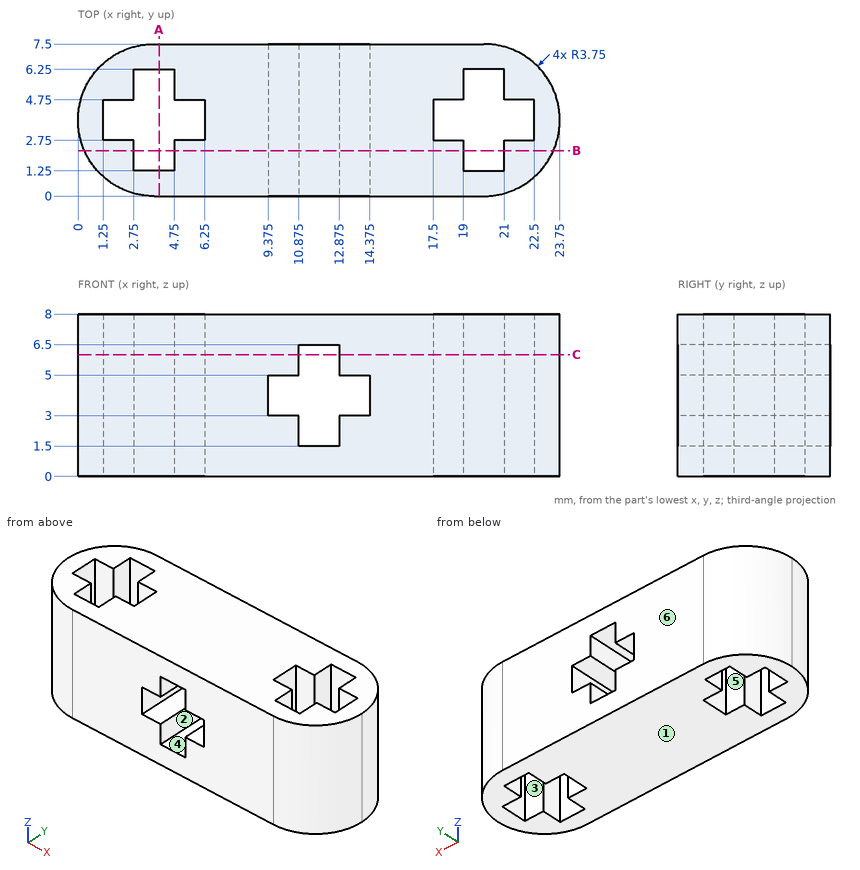
Study the drawing (mm; zero at the part's minimum x, y, z) and answer. A direction names the side the tool comes from. Give positions to 0.01 mm unless a question says otherwise; leave off trailing zeros. Order: outer loops, then holes, each group sorted by start corner. A loop starts at its lowest first (then second) coordinate and runs counter-clockwise, first axis right, second up. Notation, with made-up numbers: (11, 37.25) - (51, 37.25) arc R35 ccw to (51, 69.25) - close; hole circle Ø9 at (-30.5, 70). An arc over 180 degrees is marked (long way). Answer in a Markdown table with one row per item. Add a question column.
Q1. Find the intervals of material crossed by line 1 along Z through (x, y) = (10.5, 3.25); line 2 along X through (y, z) = (5, 0.75); line 3 along Z through (x, y) = (12, 5.75), in increasing order. Write a range as [from, to].
Q2. The part is cut by section C-C (z = 6). Give the number of separate pieces and of enclosed holes in the cut face, then the cut area to 3 significant figures.
Q3. The part is cut by section B-B (y = 2.25). Determine the outline of the cut face in (x, z) (3 decimals), then the cut area to 3 significant figures.
Q4. For a pull along Z with two mould halves and no side action, classify the marked faces 1, 2 and 3 as released by +Z, released by -Z, zero draft, split by the parting line, or undercut.
Q5. The part is cut by section A-A (x = 4). Determine the outline of the cut face in (y, z).
Q6. Given P1, Ø1.2, axis at y = 2.5, z = 3, coming from the -X side; P2, Ø1.2, axis at y = 4, z = 2, coming from the -X side; P3, Ø1.2, axis at y = 5.5, z = 2.5, coming from the +X side; P4, Ø1.7, axis at x = 2, z = 3.5, coming from the -Y side, each flat-ended and moving along its own axis, determine where each tip first touches the part or whether it passes through.
Q7. Which of the six approach directions +Z, -Z, +X, -X, +Y, -Y give full straight-line access (tool end or side, diameter ignored) to the marked faces 4, 5 and 6?
Determined:
| question | item | result |
|---|---|---|
| 1 | line 1 | z = [0, 3], [5, 8] |
| 1 | line 2 | x = [0.21, 2.75], [4.75, 19], [21, 23.54] |
| 1 | line 3 | z = [0, 1.5], [6.5, 8] |
| 2 | separate pieces | 2 |
| 2 | enclosed holes | 2 |
| 2 | area | 119 mm² |
| 3 | outline | (0.313, 0) - (2.75, 0) - (2.75, 8) - (0.313, 8) - close; (4.75, 0) - (19, 0) - (19, 8) - (4.75, 8) - close; (21, 0) - (23.437, 0) - (23.437, 8) - (21, 8) - close; hole (9.375, 3) - (10.875, 3) - (10.875, 1.5) - (12.875, 1.5) - (12.875, 3) - (14.375, 3) - (14.375, 5) - (12.875, 5) - (12.875, 6.5) - (10.875, 6.5) - (10.875, 5) - (9.375, 5) - close |
| 3 | area | 137 mm² |
| 4 | face 1 | released by -Z |
| 4 | face 2 | undercut |
| 4 | face 3 | zero draft |
| 5 | outline | (0, 0) - (1.25, 0) - (1.25, 8) - (0, 8) - close; (6.25, 0) - (7.5, 0) - (7.5, 8) - (6.25, 8) - close |
| 6 | P1 | stops at x = 0.06 |
| 6 | P2 | stops at x = 0 |
| 6 | P3 | stops at x = 23.57 |
| 6 | P4 | stops at y = 0.11 |
| 7 | face 4 | +Y, -Y |
| 7 | face 5 | +Z, -Z |
| 7 | face 6 | +Z, -Z, +X, -X, +Y |
